Geometry check sheet. Reference: drawing and pictorial views, mm from the part's lowest x, y, z. Round coordinates to 2 decimals unless told otherwise and drop trailing zeros. Write each loop counter-clockwise with the first axis right and the second up, starting at its lowest first coordinate (ties: lowest second). Pieces come first, ordered by that corner, then holes. Notation, with made-up numbers: (24.25, 25.25) - (81.25, 25.25) arc R12 cw to (81.25, 47.25) - close; hole circle Ø4 at (27, 72.5). An arc over 180 degrees is marked (long way). Use one line per item in the form item = value. Start each with the question number.
1) Section check A-A (x = 12). Record the boundary of the cut face in (y, z).
2) Draft check along X on the marked faces 1, 2, 3 and 4. Enter one of: +X half, -X half, draft (parallel to the pull), parting line (faces both ways), or undercut.
3) Section check B-B (z = 24). Record the boundary of the cut face in (x, y).
4) Gauge pin test, flat ends, axial feed: P1, Ø3, axis at y = 2.5, z = 17, coming from the -X side; P2, Ø4.5, axis at x = 12, z = 24, coming from the +Y side. Record the tip position at first contact, or that the pin passes through.
5) Section check D-D (x = 17). Record the boundary of the cut face in (y, z), then the cut area to 3 significant figures.
6) Section check C-C (z = 30.5). Record the boundary of the cut face in (x, y).
7) Scan lines: probe 1 along Z at (x, y) = (12, 3.35); probe 2 along X at (y, z) = (2, 24); probe 3 along Y at (x, z) = (15, 28). Record each from-to range of solid material in increasing order.
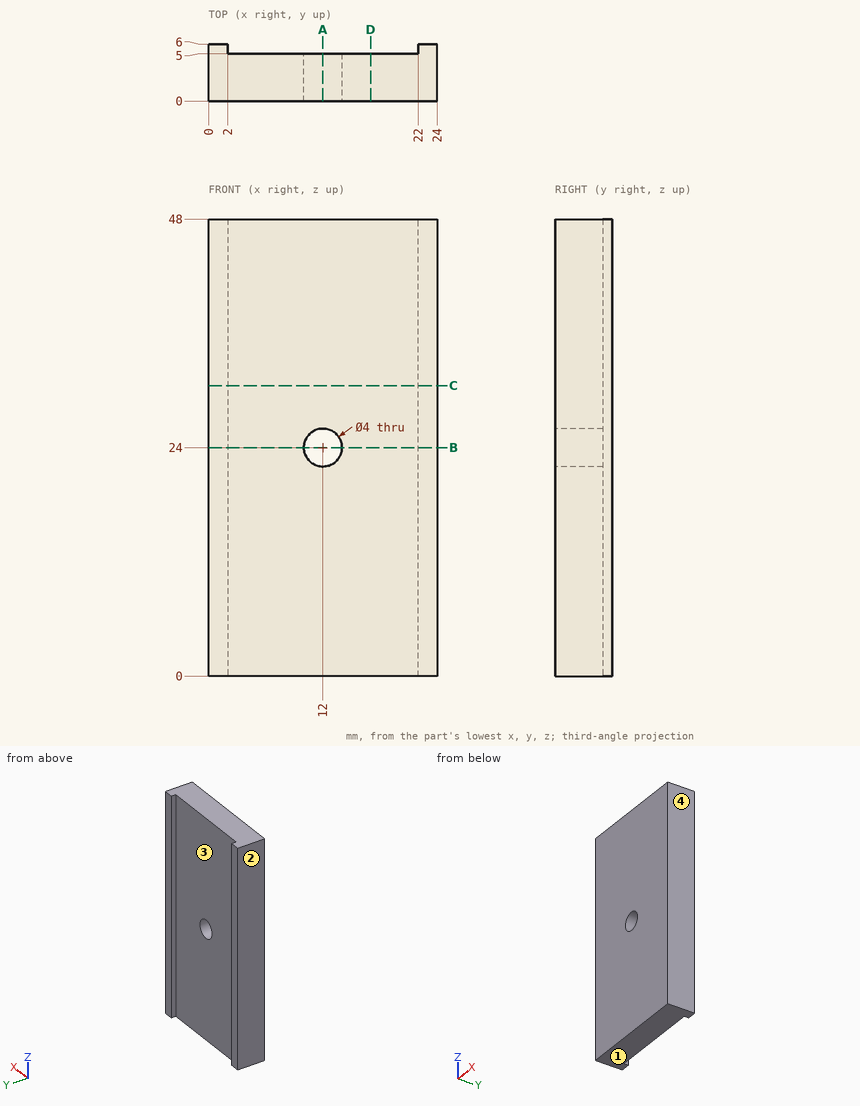
Results are:
q1.outline = (0, 0) - (5, 0) - (5, 22) - (0, 22) - close; (0, 26) - (5, 26) - (5, 48) - (0, 48) - close
q2.face_1 = draft
q2.face_2 = -X half
q2.face_3 = undercut
q2.face_4 = +X half
q3.outline = (0, 0) - (10, 0) - (10, 5) - (2, 5) - (2, 6) - (0, 6) - close; (14, 0) - (24, 0) - (24, 6) - (22, 6) - (22, 5) - (14, 5) - close
q4.P1 = 0
q4.P2 = 5
q5.outline = (0, 0) - (5, 0) - (5, 48) - (0, 48) - close
q5.area = 240 mm²
q6.outline = (0, 0) - (24, 0) - (24, 6) - (22, 6) - (22, 5) - (2, 5) - (2, 6) - (0, 6) - close
q7.probe_1 = 0 to 22, 26 to 48
q7.probe_2 = 0 to 10, 14 to 24
q7.probe_3 = 0 to 5
